Here's the drawing with two shaded views (mm, measured from the low corner). I have some questions. Round coordinates to 2 decimals unless told otherwise and drop trailing zeros. Loops run counter-clockwise (first coordinate to the right, second up) from the corner with the lowest first, then second, coordinate; pieces in that order, holes last. Notation, with made-up numbers: (59.25, 44.5) -> (63.25, 44.5) arc R24 ccw to (63.25, 82.5) -> close; hole circle Ø7 at (29.5, 54.25). An arc over 180 degrees is marked (long way). Use a Markdown table: item, result.
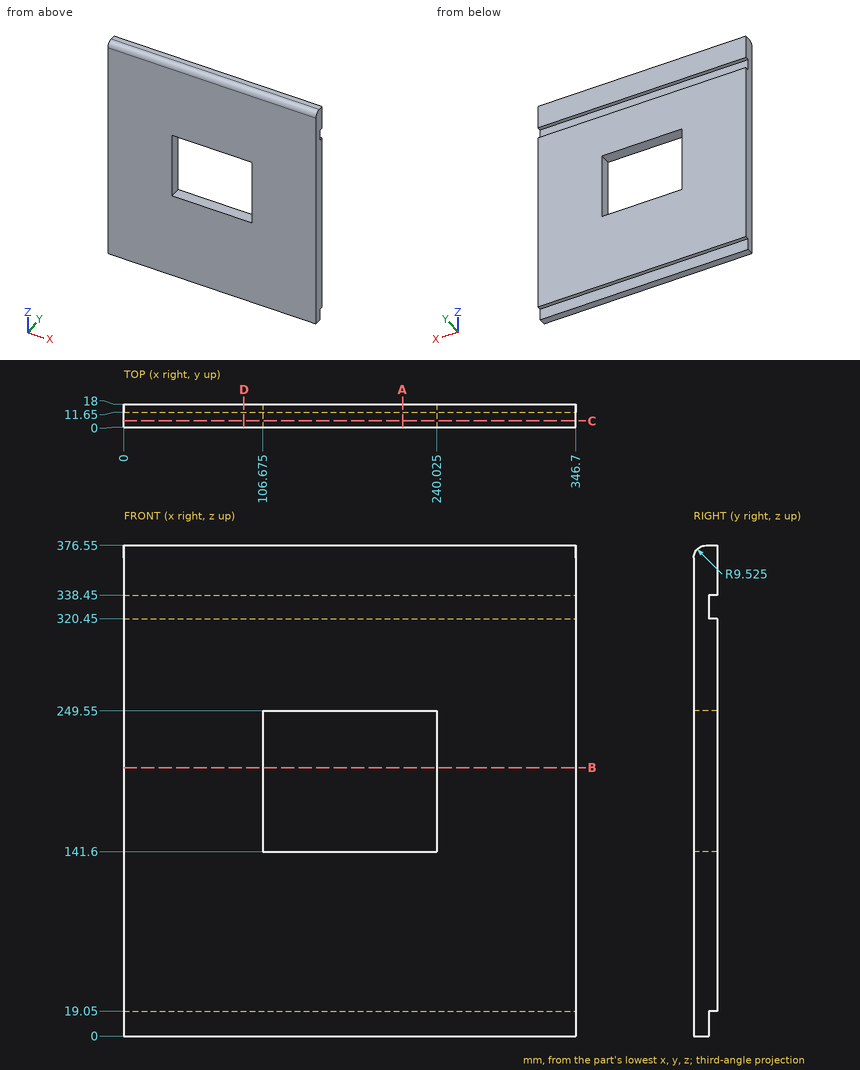
1. I need wall thicknesses on line 1 (Z direction, x = 143, y = 16.5); line 2 (X direction, y = 7.25, z = 178.5) (3 decimals); line 3 (Z direction, x = 149, y = 9.5). Which ranges of each line are inside material? Lowest first, please.
Answer sheet:
| item | result |
|---|---|
| line 1 | z = 19.05 to 141.6, 249.55 to 320.45, 338.45 to 376.55 |
| line 2 | x = 0 to 106.675, 240.025 to 346.7 |
| line 3 | z = 0 to 141.6, 249.55 to 376.55 |
2. I want a section at C-C (y = 5). Please give me the cut outline in (x, z) (3 decimals).
Answer sheet:
| item | result |
|---|---|
| outline | (0, 0) -> (346.7, 0) -> (346.7, 375.407) -> (0, 375.407) -> close; hole (106.675, 141.6) -> (240.025, 141.6) -> (240.025, 249.55) -> (106.675, 249.55) -> close |
3. I want a section at D-D (x = 92). Please give me the cut outline in (y, z) (3 decimals), plus the area to 3 significant figures.
Answer sheet:
| item | result |
|---|---|
| outline | (0, 0) -> (11.65, 0) -> (11.65, 19.05) -> (18, 19.05) -> (18, 320.45) -> (11.65, 320.45) -> (11.65, 338.45) -> (18, 338.45) -> (18, 376.55) -> (9.525, 376.55) arc R9.525 ccw to (0, 367.025) -> close |
| area | 6,520 mm² |
4. I want a section at A-A (x = 214). Please give me the cut outline in (y, z) (3 decimals), plus the area to 3 significant figures.
Answer sheet:
| item | result |
|---|---|
| outline | (0, 0) -> (11.65, 0) -> (11.65, 19.05) -> (18, 19.05) -> (18, 141.6) -> (0, 141.6) -> close; (0, 249.55) -> (18, 249.55) -> (18, 320.45) -> (11.65, 320.45) -> (11.65, 338.45) -> (18, 338.45) -> (18, 376.55) -> (9.525, 376.55) arc R9.525 ccw to (0, 367.025) -> close |
| area | 4,580 mm² |
5. I want a section at B-B (z = 206). Please give me the cut outline in (x, y) (3 decimals).
Answer sheet:
| item | result |
|---|---|
| outline | (0, 0) -> (106.675, 0) -> (106.675, 18) -> (0, 18) -> close; (240.025, 0) -> (346.7, 0) -> (346.7, 18) -> (240.025, 18) -> close |
6. Will these pins go through, and if not, where does the flat tip stop? pin 1 Ø5 at (x, y) = (65.5, 5) entering from +Z; pin 2 Ø8 at (x, y) = (268, 3) entering from +Z; pin 3 Ø7 at (x, y) = (127.5, 14) entering from -Z; pin 4 Ø1.5 at (x, z) = (142, 322.5) entering from +Y.
Answer sheet:
| item | result |
|---|---|
| pin 1 | stops at z = 376.33 |
| pin 2 | stops at z = 376.21 |
| pin 3 | stops at z = 0 |
| pin 4 | stops at y = 11.65 |
